```python
from build123d import *

# Parameters (mm, degrees)
F0_W      = 76.2
F0_H      = 101.6
F1_DEPTH  = 3.175
F2_R      = 6.35
F3_DEPTH  = 12.7
F4_R      = 3.96875
F5_R      = 3.96875
F6_DEPTH  = 38.1
F7_R      = 3.175
F7_R_2    = 3.1115
F8_DEPTH  = 25.4
F9_R      = 9.525
F9_R_2    = 6.35
F10_DEPTH = 6.35


with BuildPart() as f1:
    # F0 (on Top) → F1 (new body)
    with BuildSketch(Plane.XY):
        Rectangle(F0_W, F0_H)
    extrude(amount=F1_DEPTH)

    # F2 (on face) → F3 (join)
    with BuildSketch(Plane.XY.offset(3.175)):
        with Locations((0, 25.4)):
            Circle(F2_R)
        with Locations((0, -25.4)):
            Circle(F2_R)
    extrude(amount=F3_DEPTH)

    # F4 (on face) + F5 (on face) → F6 (cut)
    with BuildSketch(Plane.XY.offset(15.875)):
        with Locations((0, 25.4)):
            Circle(F4_R)
    with BuildSketch(Plane.XY.offset(15.875)):
        with Locations((0, -25.4)):
            Circle(F5_R)
    extrude(amount=-F6_DEPTH, mode=Mode.SUBTRACT)

    # F7 (on face) → F8 (cut)
    with BuildSketch(Plane.XY.offset(3.175)):
        with Locations((25.4, 25.4)):
            Circle(F7_R)
        with Locations((25.4, -25.4)):
            Circle(F7_R)
        with Locations((-25.4, 25.4)):
            Circle(F7_R_2)
        with Locations((-25.4, -25.4)):
            Circle(F7_R_2)
    extrude(amount=-F8_DEPTH, mode=Mode.SUBTRACT)

    # F9 (on face) → F10 (join)
    with BuildSketch(Plane.XY.offset(3.175)):
        with Locations((0, 25.4)):
            Circle(F9_R)
        with Locations((0, 25.4)):
            Circle(F9_R_2, mode=Mode.SUBTRACT)
        with Locations((0, -25.4)):
            Circle(F9_R)
        with Locations((0, -25.4)):
            Circle(F9_R_2, mode=Mode.SUBTRACT)
    extrude(amount=F10_DEPTH)


solid = f1.part
```
The model under review builds one solid part; all positions refer to its coordinate system, in mm. A direction names the side the tool comes from. Round coordinates to 2 decimals unless told otherwise and drop trailing zeros. Loops run counter-clockwise (first coordinate to the right, second up) from the corner with the lowest first, then second, coordinate; pieces in that order, holes last.
1) Consider section D-D on x = 0. State the section outline as (y, z) points (3 decimals).
Values follow:
outline: (-50.8, 0) - (-29.369, 0) - (-29.369, 15.875) - (-31.75, 15.875) - (-31.75, 9.525) - (-34.925, 9.525) - (-34.925, 3.175) - (-50.8, 3.175) - close; (-21.431, 0) - (21.431, 0) - (21.431, 15.875) - (19.05, 15.875) - (19.05, 9.525) - (15.875, 9.525) - (15.875, 3.175) - (-15.875, 3.175) - (-15.875, 9.525) - (-19.05, 9.525) - (-19.05, 15.875) - (-21.431, 15.875) - close; (29.369, 0) - (50.8, 0) - (50.8, 3.175) - (34.925, 3.175) - (34.925, 9.525) - (31.75, 9.525) - (31.75, 15.875) - (29.369, 15.875) - close
2) Clearance check with flat-ended pins moving along their axes: P1, Ø21, axis at x = -1.5, y = 28, coming from the +Z side (3 decimals); P2, Ø5, axis at x = 1, z = 10, coming from the -Y side (3 decimals); P3, Ø3, axis at x = -3.5, z = 8, coming from the +Y side; P4, Ø5, axis at x = 25.4, y = -25.4, coming from the +Z side. State where each tip first meets the part, or that it passes through.
Values follow:
P1: stops at z = 15.875
P2: stops at y = -34.925
P3: stops at y = 34.71
P4: passes through
3) The part is to be moulded in two halves that separate along X. For faces 1 (the face through (28.43, 26.35, 1.61)), 2 (the face through (5.12, -17.37, 6.31)), 3 (the face through (-1, -50.8, 2)), say which applies: pulls with the +X half, pulls with the -X half, needs draft (parallel to the pull), parting line crosses it, or undercut.
Values follow:
face 1: undercut
face 2: parting line crosses it
face 3: needs draft
4) Consider section B-B on x = -25.4. State the section outline as (y, z) points (1 decimal), then the cut area to 3 significant figures.
Values follow:
outline: (-50.8, 0) - (-28.5, 0) - (-28.5, 3.2) - (-50.8, 3.2) - close; (-22.3, 0) - (22.3, 0) - (22.3, 3.2) - (-22.3, 3.2) - close; (28.5, 0) - (50.8, 0) - (50.8, 3.2) - (28.5, 3.2) - close
area: 283 mm2
5) Consider section A-A on y = -25.4. Give the number of separate pieces and of enclosed holes in the cut face, then the cut area to 3 significant figures.
Values follow:
separate pieces: 4
enclosed holes: 0
area: 278 mm2
6) Wall thickness on line 1 along Y through (x, z) = (0, 5) (3 decimals); line 2 along Y through (x, z) = (25.4, 1.7) (3 decimals); line 3 along Y through (x, z) = (3, 12.5): over which ranges is each line inside the solid? List them lowest first.
Values follow:
line 1: y = -34.925 to -29.369, -21.431 to -15.875, 15.875 to 21.431, 29.369 to 34.925
line 2: y = -50.8 to -28.575, -22.225 to 22.225, 28.575 to 50.8
line 3: y = -31 to -28, -22.8 to -19.8, 19.8 to 22.8, 28 to 31
7) Tool access review of faces 4 (the face through (-1, 1, 0)), 5 (the face through (2.93, 19.766, 12.656)): name each direction out of +Z, -Z, +X, -X, +Y, -Y from which nothing blocks a thin tool from reaching the whole face with its end or side.
Values follow:
face 4: -Z, +X, -X, +Y, -Y
face 5: +Z
